Geometry: final body of the model. Coordinates: model frame, mm. Face numbers are marked on the shaded views. A direction names the side the tool comes from. Round coordinates to 2 decimals unless told otherwise and drop trailing zeros. Write each loop counter-clockwise with the first axis right and the second up, starting at its lowest first coordinate (ties: lowest second). Pieces come first, ordered by that corner, then holes. Notation, with made-up numbers: M 10.25,47.5 L 56.25,47.5 A12 cw 56.25,69.5 Z; hole C 47,62 d9. An arc over 180 degrees is marked long. Put each result on its own line as item: value. Start each with the question number.
```python
from build123d import *

# Parameters (mm, degrees)
F0_R     = 1.9685
F1_DEPTH = 3.4544
F2_W     = 1.9558
F2_H     = 0.9525
F3_DEPTH = 16.7142
F4_R     = 4.572
F6_DEPTH = 9.399
F7_R     = 0.254
F8_SIZE2 = 0.5719231767
F8_SIZE  = 0.3302


with BuildPart() as f1:
    # F0 (on Top) → F1 (new body)
    with BuildSketch(Plane.XY):
        Polygon((-7.9248, 5.9309), (-7.9248, -5.9309), (2.8448, -5.9309), (2.8448, -3.4671), (8.7884, -3.4671), (8.7884, 5.9309), align=None)
        Circle(F0_R, mode=Mode.SUBTRACT)
    extrude(amount=-F1_DEPTH)

    # F2 (on face) → F3 (cut, through all)
    with BuildSketch(Plane(origin=(-7.9248, 0, 0), x_dir=(0, -1, 0), z_dir=(-1, 0, 0))):
        with Locations((-4.953, -0.47625)):
            Rectangle(F2_W, F2_H)
        with Locations((4.953, -0.47625)):
            Rectangle(F2_W, F2_H)
    extrude(amount=-F3_DEPTH, mode=Mode.SUBTRACT)

    # F4
    f4_edges = [f1.edges().sort_by_distance(p)[0] for p in [
        (-7.9248, -5.9309, -2.20345),
        (-7.9248, 5.9309, -2.20345),
    ]]
    fillet(f4_edges, radius=F4_R)

    # F5 (on face) → F6 (cut, through all)
    with BuildSketch(Plane.XZ.offset(3.4671)):
        with BuildLine():
            ThreePointArc((6.417348453, 0), (7.7501634134, -0.858086307), (8.7884, -2.0559062515))
            Line((8.7884, -2.0559062515), (8.7884, 0))
            Line((8.7884, 0), (6.417348453, 0))
        make_face()
    extrude(amount=-F6_DEPTH, mode=Mode.SUBTRACT)

    # F7
    f7_edges = [f1.edges().sort_by_distance(p)[0] for p in [
        (-2.128745, -3.9751, 0),
        (-0.342471, 3.9751, 0),
        (-2.128745, -3.9751, -0.9525),
        (0.377001, 3.9751, -0.9525),
    ]]
    fillet(f7_edges, radius=F7_R)

    # F8
    f8_edges = [f1.edges().sort_by_distance(p)[0] for p in [
        (-1.9685, 0, -3.4544),
    ]]
    f8_side = f1.faces().sort_by_distance((2.7178, 5.725953, -3.4544))[0]
    chamfer(f8_edges, length=F8_SIZE, length2=F8_SIZE2, reference=f8_side)


solid = f1.part
```
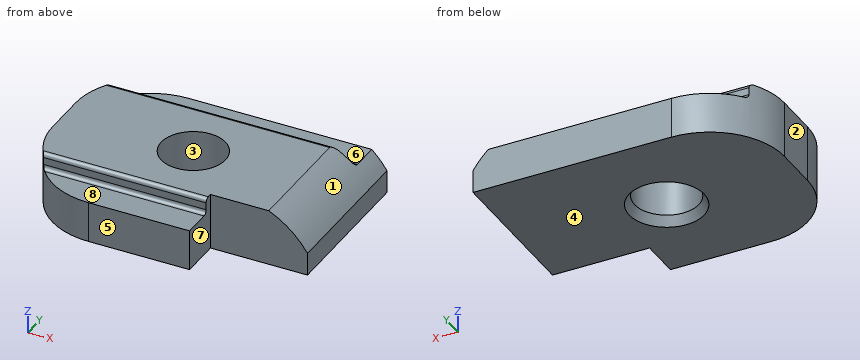
1) Ray query, probe 1 along Y at (x, z) = (0, -2); probe 2 along Z at (x, y) = (-1.75, 4.75); probe 3 along X at (y, z) = (0.25, -1.85). Return the intervals inside material, ascending.
2) Access query for the marked faces 5, 6, 7 and 8. Directions: +Z, -Z, +X, -X, +Y, -Y. A direction counts if a zero-diameter tool reaches every point of the face in a straight line with its end or side. Return the directions, or none.
3) Section D-D, the plane x = 5.75. Output: boundary loops of the cut face in (y, z).
4) Section C-C, the plane z = -2.4. Output: boundary loops of the cut face in (x, y), and give its area (3 significant figures).
5) Draft query along X for the marked faces 1, 2, 3 and 4. Return one class per face: +X half, -X half, draft (parallel to the pull), parting line (faces both ways), or undercut.
6) Section A-A, the plane x = 0. Output: boundary loops of the cut face in (y, z).
7) Section B-B, the plane y = 0. Output: boundary loops of the cut face in (x, z), and give its area (3 significant figures).
8) First-contact query: pin 1 (0.5 mm diameter, centred on x = -1.5, y = -5, fed in from +Z); pin 2 (2 mm diameter, centred on y = 2.5, z = -0.5, fed in from -X). Flat tips, straight axial feed; report the tip coordinate or a pass-through.
Solved:
1. probe 1: y = -5.93 to -1.97, 1.97 to 5.93
1. probe 2: z = -3.45 to -0.95
1. probe 3: x = -7.92 to -1.95, 1.95 to 8.65
2. face 5: +Z, -Z, +X, -X, -Y
2. face 6: +Z, +X, -X, +Y
2. face 7: +Z, -Z, +X, -Y
2. face 8: +Z, +X, -X, -Y
3. outline: M -3.47,-3.45 L 5.93,-3.45 L 5.93,-0.95 L 4.23,-0.95 A0.25 cw 3.98,-0.7 L 3.98,-0.25 A0.25 ccw 3.72,0 L -3.47,0 Z
4. outline: M -7.92,-1.36 A4.57 ccw -3.35,-5.93 L 2.84,-5.93 L 2.84,-3.47 L 8.79,-3.47 L 8.79,5.93 L -3.35,5.93 A4.57 ccw -7.92,1.36 Z; hole C 0,0 d3.94
4. area: 162 mm2
5. face 1: +X half
5. face 2: -X half
5. face 3: undercut
5. face 4: draft
6. outline: M -5.93,-3.45 L -2.3,-3.45 L -1.97,-2.88 L -1.97,0 L -3.72,0 A0.25 ccw -3.98,-0.25 L -3.98,-0.7 A0.25 cw -4.23,-0.95 L -5.93,-0.95 Z; M 1.97,-2.88 L 2.3,-3.45 L 5.93,-3.45 L 5.93,-0.95 L 4.23,-0.95 A0.25 cw 3.98,-0.7 L 3.98,-0.25 A0.25 ccw 3.72,0 L 1.97,0 Z
7. outline: M -7.92,-3.45 L -2.3,-3.45 L -1.97,-2.88 L -1.97,0 L -7.92,0 Z; M 1.97,-2.88 L 2.3,-3.45 L 8.79,-3.45 L 8.79,-2.06 A5.59 ccw 6.42,0 L 1.97,0 Z
7. area: 42.0 mm2
8. pin 1: stops at z = -0.95
8. pin 2: stops at x = -7.92
